Read the model definition and answer for the solid it produces. Units are mm, in the model's axes. Round coordinates to 2 decimals unless told otherwise and drop trailing zeros. Order: outer loops, then holes, each group sorted by start corner. A loop starts at its lowest first (then second) coordinate and runs counter-clockwise, first axis right, second up. Notation, with made-up numbers: M -39.75,84.5 L 3.25,84.5 A26 ccw 3.25,105.5 Z; hole C -23.5,48 d10. An arc over 180 degrees is marked long. Answer as CSV lines item,"result".
```python
from build123d import *

# Parameters (mm, degrees)
SKETCH1_R           = 75
SKETCH1_R_2         = 4.25
BOSS_EXTRUDE1_DEPTH = 5.5
SKETCH4_R           = 2.625
CUT_EXTRUDE2_DEPTH  = 5.5
CUT_EXTRUDE3_DEPTH  = 5.5


with BuildPart() as part:
    # Sketch1 → Boss-Extrude1 (new body)
    with BuildSketch(Plane(origin=(0, 0, 0), x_dir=(1, 0, 0), z_dir=(0, 1, 0))):
        with Locations(Location((0, 0, 0), (0, 0, 270))):
            Circle(SKETCH1_R)
        with Locations(Location((0, 0, 0), (0, 0, 270))):
            Circle(SKETCH1_R_2, mode=Mode.SUBTRACT)
    extrude(amount=BOSS_EXTRUDE1_DEPTH)

    # Sketch4 → Cut-Extrude2 (cut)
    with BuildSketch(Plane(origin=(0, 5.5, 0), x_dir=(1, 0, 0), z_dir=(0, 1, 0))):
        with Locations(Location((44.547727215, -44.547727215, 0), (0, 0, 270))):
            Circle(SKETCH4_R)
        with Locations(Location((-44.547727215, -44.547727215, 0), (0, 0, 270))):
            Circle(SKETCH4_R)
        with Locations(Location((44.547727215, 44.547727215, 0), (0, 0, 270))):
            Circle(SKETCH4_R)
        with Locations(Location((-44.547727215, 44.547727215, 0), (0, 0, 270))):
            Circle(SKETCH4_R)
        Polygon((7.794228634, 0), (3.897114317, 6.75), (-3.897114317, 6.75), (-7.794228634, 0), (-3.897114317, -6.75), (3.897114317, -6.75), align=None)
    extrude(amount=-CUT_EXTRUDE2_DEPTH, mode=Mode.SUBTRACT)

    # Sketch5 → Cut-Extrude3 (cut)
    with BuildSketch(Plane(origin=(0, 5.5, 0), x_dir=(1, 0, 0), z_dir=(0, 1, 0))):
        with BuildLine():
            Line((32, -17), (48.083261121, -17))
            ThreePointArc((48.083261121, -17), (36.062445841, -36.062445841), (17, -48.083261121))
            Line((17, -48.083261121), (17, -32))
            ThreePointArc((17, -32), (21.393398282, -21.393398282), (32, -17))
        make_face()
        with BuildLine():
            Line((-17, -32), (-17, -48.083261121))
            ThreePointArc((-17, -48.083261121), (-36.062445841, -36.062445841), (-48.083261121, -17))
            Line((-48.083261121, -17), (-32, -17))
            ThreePointArc((-32, -17), (-21.393398282, -21.393398282), (-17, -32))
        make_face()
        with BuildLine():
            Line((17, 32), (17, 48.083261121))
            ThreePointArc((17, 48.083261121), (36.062445841, 36.062445841), (48.083261121, 17))
            Line((48.083261121, 17), (32, 17))
            ThreePointArc((32, 17), (21.393398282, 21.393398282), (17, 32))
        make_face()
        with BuildLine():
            Line((-32, 17), (-48.083261121, 17))
            ThreePointArc((-48.083261121, 17), (-36.062445841, 36.062445841), (-17, 48.083261121))
            Line((-17, 48.083261121), (-17, 32))
            ThreePointArc((-17, 32), (-21.393398282, 21.393398282), (-32, 17))
        make_face()
    extrude(amount=-CUT_EXTRUDE3_DEPTH, mode=Mode.SUBTRACT)


solid = part.part
```
Item 1: A cutting plane is placed at C-C, the plane x = 37. Determine the outline of the cut face in (y, z).
Ans:
outline,"M 0,-65.24 L 5.5,-65.24 L 5.5,-35.1 L 0,-35.1 Z; M 0,-17 L 5.5,-17 L 5.5,17 L 0,17 Z; M 0,35.1 L 5.5,35.1 L 5.5,65.24 L 0,65.24 Z"
Item 2: Determine the mould class of faces 1 (the face through (0, 3, 6.75)), 2 (the face through (-16, 5.5, -1)) for opening direction Z: +Z half, -Z half, draft (parallel to the pull), parting line (faces both ways), or undercut.
Ans:
face 1,"undercut"
face 2,"draft"
Item 3: A cutting plane is placed at A-A, the plane z = 25.5. Determine the outline of the cut face in (x, y).
Ans:
outline,"M -70.53,0 L -44.17,0 L -44.17,5.5 L -70.53,5.5 Z; M -18.48,0 L 18.48,0 L 18.48,5.5 L -18.48,5.5 Z; M 44.17,0 L 70.53,0 L 70.53,5.5 L 44.17,5.5 Z"
Item 4: Find the intervals of material crossed by probe 1 along Z at (x, y) = (-33, 5.2); probe 2 along Z at (x, y) = (22, 1.4); probe 3 along X at (y, z) = (1.3, 45), in increasing order. Write a range as [from, to].
Ans:
probe 1,"[-67.35, -38.88], [-17, 17], [38.88, 67.35]"
probe 2,"[-71.7, -46.01], [-20.82, 20.82], [46.01, 71.7]"
probe 3,"[-60, -47.13], [-41.96, -24], [-17, 17], [24, 41.96], [47.13, 60]"
Item 5: Flat-ended cylindrical pins translate along their axes: pin 1 (1.6 mm diameter, centred on x = 1, y = 2.5, fed in from +Z); pin 2 (4.5 mm diameter, centred on x = 44.55, z = -44.55, fed in from +Y); pin 3 (1.6 mm diameter, centred on x = -38, y = 3.5, fed in from -Z); pin 4 (3 mm diameter, centred on x = -41, y = 2.5, fed in from +Z). Find the tip coordinate at first contact, or state that the pin passes through.
Ans:
pin 1,"z = 75"
pin 2,"through"
pin 3,"z = -65.12"
pin 4,"z = 63.76"
Item 6: A cutting plane is placed at D-D, the plane y = 1. Give the number of separate pieces and of enclosed holes in the cut face, and give its area (3 significant figures).
Ans:
separate pieces,"1"
enclosed holes,"9"
area,"15,100 mm2"
Item 7: A cutting plane is placed at B-B, the plane x = 0. Determine the outline of the cut face in (y, z).
Ans:
outline,"M 0,-75 L 5.5,-75 L 5.5,-6.75 L 0,-6.75 Z; M 0,6.75 L 5.5,6.75 L 5.5,75 L 0,75 Z"
